Autodesk Inventor part; units mm, degrees
ref_plane "YZ Plane" through (0, 0, 0) normal (1, 0, 0) x (0, 1, 0)
ref_plane "XZ Plane" through (0, 0, 0) normal (0, 1, 0) x (-1, 0, 0)
ref_plane "XY Plane" through (0, 0, 0) normal (0, 0, 1) x (1, 0, 0)
sketch "Sketch1" plane through (0, 0, 0) normal (0, 0, 1) x (1, 0, 0)
  line L0 (0, 0) -> (96.8375, 0)
  line L1 (96.8375, 0) -> (96.8375, 41.275)
  line L2 (96.8375, 41.275) -> (0, 41.275)
  line L3 (0, 41.275) -> (0, 0)
  circle A0 centre (87.3125, 31.75) radius 7.112
  circle A1 centre (76.2, 31.75) radius 2.3241
  circle A2 centre (65.0875, 31.75) radius 3.3274
  circle A3 centre (42.8625, 31.75) radius 3.9624
  circle A4 centre (31.75, 31.75) radius 3.9624
  point P0 (9.525, 9.525)
  point P1 (9.525, 20.6375)
  point P2 (9.525, 31.75)
  point P3 (20.6375, 9.525)
  point P4 (20.6375, 20.6375)
  point P5 (20.6375, 31.75)
  point P6 (31.75, 9.525)
  point P7 (31.75, 20.6375)
  point P8 (42.8625, 9.525)
  point P9 (42.8625, 20.6375)
  point P10 (53.975, 9.525)
  point P11 (53.975, 20.6375)
  point P12 (53.975, 31.75)
  point P13 (65.0875, 9.525)
  point P14 (65.0875, 20.6375)
  point P15 (76.2, 9.525)
  point P16 (76.2, 20.6375)
  point P17 (87.3125, 9.525)
  point P18 (87.3125, 20.6375)
  dimension "d0" = 9.525
  dimension "d2" = 9.525
  dimension "d5" = 11.1125
  dimension "d8" = 11.1125
  dimension "d11" = 9.525
  dimension "d12" = 9.525
  dimension "d50" = 14.224
  dimension "d51" = 4.6482
  dimension "d52" = 6.6548
  dimension "d53" = 7.9248
  dimension "d54" = 7.9248
extrude "Extrusion1" add sketch "Sketch1" along normal blind 3.175 contours L3 L2 L1 L0 | A0 | A1 | A2 | A3 | A4
hole "10-32" at (9.525, 9.525, 0) at (9.525, 20.6375, 0) at (9.525, 31.75, 0) at (20.6375, 9.525, 0) at (20.6375, 20.6375, 0) at (20.6375, 31.75, 0) at (31.75, 9.525, 0) at (31.75, 20.6375, 0) at (31.75, 31.75, 0) direction (0, 0, 1) diameter 3.9624 end through all
hole "8-32" at (42.8625, 31.75, 0) at (42.8625, 20.6375, 0) at (42.8625, 9.525, 0) direction (0, 0, 1) diameter 3.302 end through all
hole "6-32" at (53.975, 9.525, 0) at (53.975, 20.6375, 0) at (53.975, 31.75, 0) at (65.0875, 9.525, 0) at (65.0875, 20.6375, 0) at (65.0875, 31.75, 0) direction (0, 0, 1) diameter 2.6416 end through all
hole "4-40" at (76.2, 9.525, 0) at (76.2, 20.6375, 0) at (76.2, 31.75, 0) at (87.3125, 9.525, 0) direction (0, 0, 1) diameter 2.159 end through all
hole "1/4-20" at (87.3125, 20.6375, 0) at (87.3125, 31.75, 0) direction (0, 0, 1) diameter 4.9784 end through all
properties part number "Bolt Holder"
Work out the finished part from the listing and answer in its coordinate system (mm). Round coordinates to 2 decimals unless told otherwise and drop trailing zeros. Write each loop counter-clockwise with the first axis right and the second up, starting at its lowest first coordinate (ties: lowest second). Pieces come first, ordered by that corner, then holes.
1) A cutting plane is placed at B-B (z = 1.9). Give the number of separate pieces and of enclosed holes in the cut face, plus the area to 3 significant figures.
2) A cutting plane is placed at A-A (x = 76.2). Give the vertices of the cut face in (y, z) (1 decimal), plus the area to 3 significant figures.
3) The mould has two halves that part along Y. Classify faces 1 (the flat face through (49, 41.275, 2)), 2 (the cylindrical face through (30.08, 10.59, 1.61)), 3 (the flat face through (96.838, 20, 2)): pulls with the +Y half, pulls with the -Y half, needs draft (parallel to the pull), parting line crosses it, or undercut.
4) Given pin 1 Ø3 at (x, y) = (87.31, 20.64) entering from -Z, flat-ended and moving along its own axis, determine where the tip first touches the part or whether it passes through.
5) Straight lines are drawn through the part: line 1 (Y direction, x = 31.75, z = 1.6) (3 decimals); line 2 (Y direction, x = 43, z = 0.2) (3 decimals); line 3 (Y direction, x = 88.5, z = 2.4) (3 decimals). For each, find the intervals that lie inside material, in ascending order.
Completed:
1. separate pieces: 1
1. enclosed holes: 24
1. area: 3,770 mm2
2. outline: (0, 0) - (8.4, 0) - (8.4, 3.2) - (0, 3.2) - close; (10.6, 0) - (19.6, 0) - (19.6, 3.2) - (10.6, 3.2) - close; (21.7, 0) - (30.7, 0) - (30.7, 3.2) - (21.7, 3.2) - close; (32.8, 0) - (41.3, 0) - (41.3, 3.2) - (32.8, 3.2) - close
2. area: 110 mm2
3. face 1: pulls with the +Y half
3. face 2: undercut
3. face 3: needs draft
4. pin 1: passes through
5. line 1: y = 0 to 7.544, 11.506 to 18.656, 22.619 to 29.769, 33.731 to 41.275
5. line 2: y = 0 to 7.88, 11.17 to 18.992, 22.283 to 30.105, 33.395 to 41.275
5. line 3: y = 0 to 18.45, 22.825 to 29.562, 33.938 to 41.275
